Job drawing, mm, ordinate dimensions from the low corner. One solid piece. Round coordinates to 2 decimals unless told otherwise and drop trailing zeros. Write each loop counter-clockwise with the first axis right and the second up, starting at its lowest first coordinate (ties: lowest second). Pieces come first, ordered by that corner, then holes. Notation, with made-up numbers: (44.25, 18) - (99.25, 18) arc R30 cw to (99.25, 56) - close; hole circle Ø5 at (52.25, 68). An arc over 180 degrees is marked (long way). Write each question's results on one line, items separated by ' | '.
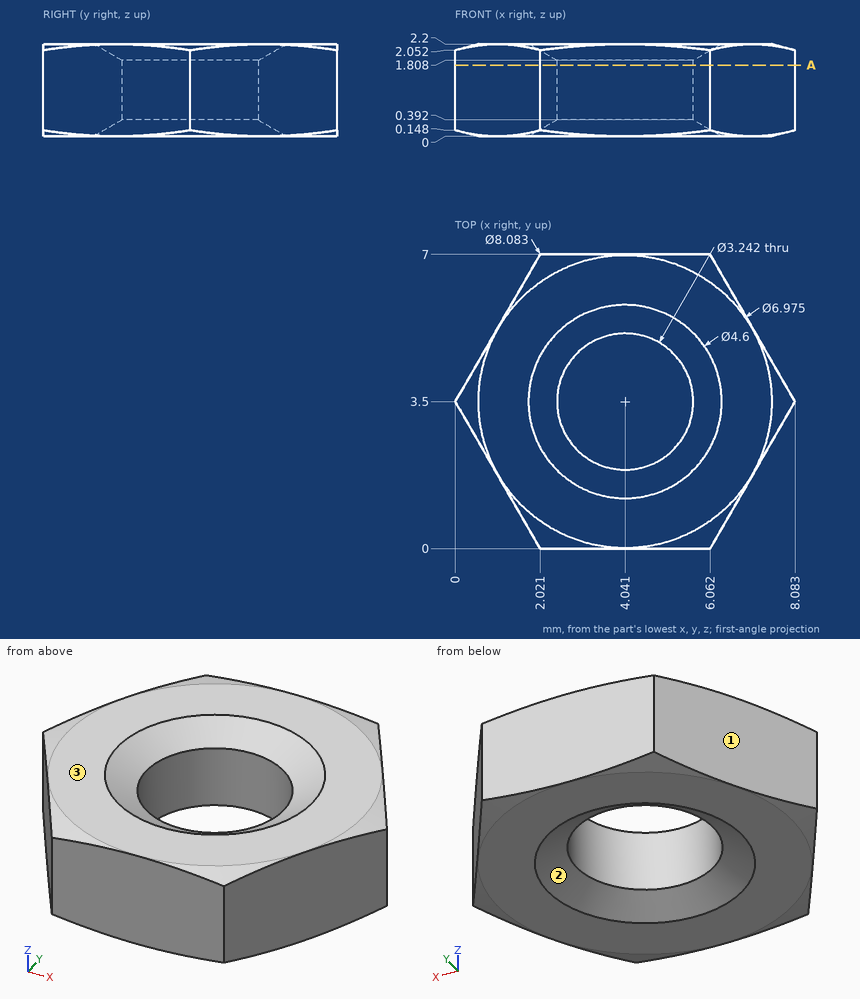
(1) Two-plate mould, pull along X, no slides. Class the marked faces 1, 2 and 3: released by +X, released by -X, zero draft, split by the parting line, or undercut.
Worked answers:
face 1: released by -X | face 2: undercut | face 3: zero draft
(2) Flat gauge pin, fed straight in: pin 1 Ø1 at (y, z) = (1.5, 1) entering from +X. Where does the tip first touch, or does it go through?
Worked answers:
pin 1: stops at x = 7.22
(3) Drill centre lines: probe 1 along Y at (x, z) = (5, 0.95) (1 decimal); probe 2 along Y at (x, z) = (3.75, 1.35) (1 decimal); probe 3 along X at (y, z) = (4.5, 0.8) (1 decimal). Where is each one in solid material? Low to high. Write a range as [from, to].
Worked answers:
probe 1: y = [0, 2.2], [4.8, 7] | probe 2: y = [0, 1.9], [5.1, 7] | probe 3: x = [0.6, 2.8], [5.3, 7.5]
(4) Slice it at A-A, the plane z = 1.7. Write the cut outline in (x, y).
Worked answers:
outline: (0, 3.5) - (2.02, 0) - (6.06, 0) - (8.08, 3.5) - (6.06, 7) - (2.02, 7) - close; hole circle Ø3.24 at (4.04, 3.5)
